The drawing under review shows one solid part. Ordinate dimensions are in mm from its lowest x, y, z. Give positions to 0.01 mm unless a question says otherwise; leave off trailing zeros. Loops run counter-clockwise (first coordinate to the right, second up) from the corner with the lowest first, then second, coordinate; pieces in that order, holes last. Notation, with made-up numbers: (67, -36.5) - (111, -36.5) arc R9 ccw to (111, -26.5) - close; hole circle Ø8 at (67, -34.5). An arc over 180 degrees is marked (long way). Write each question's results on one line, items separated by ' | '.
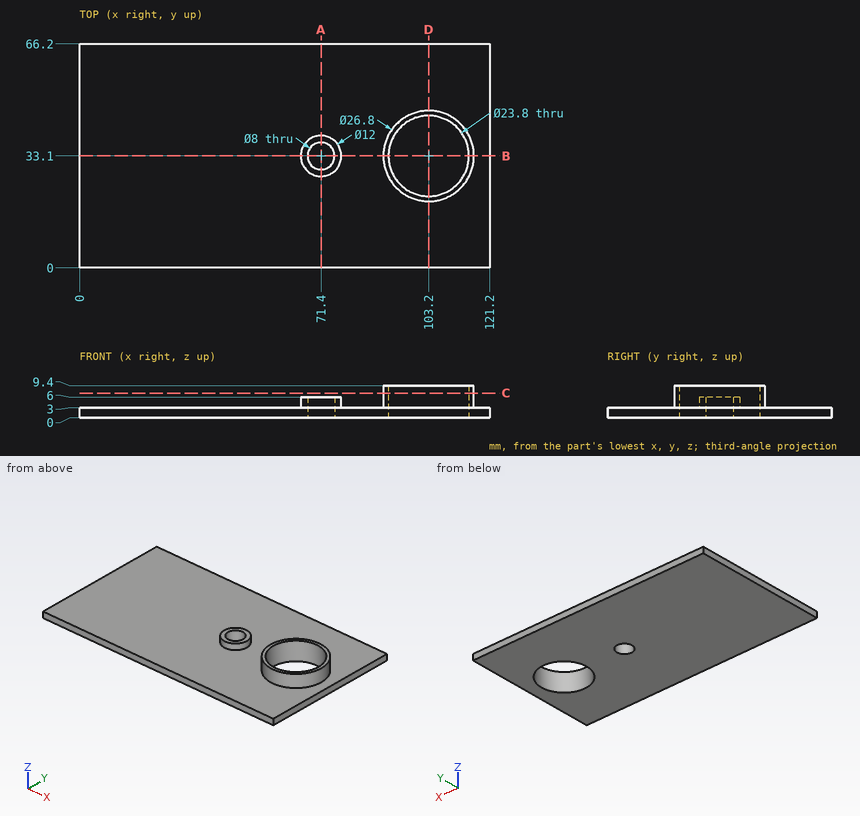
(1) Take a section at C-C on z = 7.25. Give the boundary of the cut face in (x, y), plus the area to 3 significant figures.
Answers below:
outline: circle Ø26.8 at (103.2, 33.1); hole circle Ø23.8 at (103.2, 33.1) | area: 119 mm2
(2) Take a section at A-A on x = 71.4. Give the boundary of the cut face in (y, z).
Answers below:
outline: (0, 0) - (29.1, 0) - (29.1, 6) - (27.1, 6) - (27.1, 3) - (0, 3) - close; (37.1, 0) - (66.2, 0) - (66.2, 3) - (39.1, 3) - (39.1, 6) - (37.1, 6) - close
(3) Wall thickness on line 1 along Y through (x, z) = (103.2, 5); line 2 along Y through (x, z) = (71.4, 3.9); line 3 along Z through (x, y) = (81, 56.5): over which ranges is each line inside the solid? List them lowest first. Write a range as from..to.
Answers below:
line 1: 19.7..21.2, 45..46.5 | line 2: 27.1..29.1, 37.1..39.1 | line 3: 0..3
(4) Insertion check: P1, Ø4, axis at x = 107, y = 17.5, coming from the -Z side; P2, Ø8, axis at x = 55, y = 30, coming from the +Z side; P3, Ø12, axis at x = 74.5, y = 31, coming from the +Z side. Each pin has a flat end and moves straight along its axis. Give the tip position at first contact, or say it passes through.
Answers below:
P1: z = 0 | P2: z = 3 | P3: z = 6
(5) Take a section at D-D on x = 103.2. Give the boundary of the cut face in (y, z).
Answers below:
outline: (0, 0) - (21.2, 0) - (21.2, 9.4) - (19.7, 9.4) - (19.7, 3) - (0, 3) - close; (45, 0) - (66.2, 0) - (66.2, 3) - (46.5, 3) - (46.5, 9.4) - (45, 9.4) - close
(6) Take a section at B-B on y = 33.1. Give the boundary of the cut face in (x, z), plus the area to 3 significant figures.
Answers below:
outline: (0, 0) - (67.4, 0) - (67.4, 6) - (65.4, 6) - (65.4, 3) - (0, 3) - close; (75.4, 0) - (91.3, 0) - (91.3, 9.4) - (89.8, 9.4) - (89.8, 3) - (77.4, 3) - (77.4, 6) - (75.4, 6) - close; (115.1, 0) - (121.2, 0) - (121.2, 3) - (116.6, 3) - (116.6, 9.4) - (115.1, 9.4) - close | area: 299 mm2
